The model under review builds one solid part; all positions refer to its coordinate system, in mm. Give positions to 0.01 mm unless a question says otherwise; leave off trailing zeros. Order: outer loops, then holes, each group sorted by start corner. A loop starts at its lowest first (then second) coordinate and runs counter-clockwise, first axis right, second up. Notation, with made-up numbers: (44, -1) - (99, -1) arc R9 ccw to (99, 12) - close; hole circle Ø3 at (-37.5, -21.75). An arc over 180 degrees is marked (long way). Answer as CSV lines item,"result". Start each with the question number.
Autodesk Inventor part; units mm, degrees
ref_plane "YZ Plane" through (0, 0, 0) normal (1, 0, 0) x (0, 1, 0)
ref_plane "XZ Plane" through (0, 0, 0) normal (0, 1, 0) x (-1, 0, 0)
ref_plane "XY Plane" through (0, 0, 0) normal (0, 0, 1) x (1, 0, 0)
sketch "Sketch1" plane through (0, 0, 0) normal (0, 1, 0) x (-1, 0, 0)
  circle A0 centre (0, 0) radius 3.5 construction
  line L0 (-2.0207, -3.5) -> (-4.0415, 0)
  line L1 (-4.0415, 0) -> (-2.0207, 3.5)
  line L2 (-2.0207, 3.5) -> (2.0207, 3.5)
  line L3 (2.0207, 3.5) -> (4.0415, 0)
  line L4 (4.0415, 0) -> (2.0207, -3.5)
  line L5 (2.0207, -3.5) -> (-2.0207, -3.5)
  point P0 (0, -3.5)
  dimension "d0" = 7
extrude "Extrusion1" add sketch "Sketch1" along normal mid plane 3
sketch "Sketch2" plane through (0, 1.5, 0) normal (0, 1, 0) x (1, 0, 0)
  circle A0 centre (0, 0) radius 2
  dimension "d3" = 4
extrude "Extrusion2" cut sketch "Sketch2" against normal blind 3
fillet "Fillet1" radius 0.2 12 edges at (-3.0311, 1.5, 1.75) (0, 1.5, 3.5) (3.0311, 1.5, 1.75) (3.0311, 1.5, -1.75) (0, 1.5, -3.5) (-3.0311, 1.5, -1.75) (0, -1.5, 3.5) (-3.0311, -1.5, 1.75) (-3.0311, -1.5, -1.75) (0, -1.5, -3.5) (3.0311, -1.5, -1.75) (3.0311, -1.5, 1.75)
fillet "Fillet2" radius 0.1 2 edges at (-2, 1.5, 0) (-2, -1.5, 0)
thread "Thread1"
properties part number "M4 Nut" material "Stainless Steel"
Item 1: Take a section at A-A on x = 0. Write out the cut boundary in (y, z), and give its area (3 significant figures).
Item 2: Mouldability with a two-part tool opening along X and no side actions: class faces 1 (the face through (2.993, -1.443, -1.695)), 2 (the face through (0, 0, 2)), 3 (the face through (-2, 1.5, 2)), 4 (the face through (-2.993, -1.443, 1.695)) as released by +X, released by -X, zero draft, split by the parting line, or undercut.
Item 3: Clearance check with a flat-ended pin moving along its axis: pin 1 (1.5 mm diameter, centred on x = -1, z = 0, fed in from -Y). State where the tip first meets the part, or that it passes through.
Item 4: For line 1 along Z through (x, y) = (0, -1.2); line 2 along Z through (x, y) = (-1, 1.1); line 3 along X through (y, z) = (-1.2, 0.5), list the stretches that pass through material, from the lowest coordinate up.
Item 5: Take a section at B-B on y = 0.8. Write out the cut boundary in (x, z), and give its area (3 significant figures).
Data:
1,outline,"(-1.5, -3.3) arc R0.2 ccw to (-1.3, -3.5) - (1.3, -3.5) arc R0.2 ccw to (1.5, -3.3) - (1.5, -2.1) arc R0.1 ccw to (1.4, -2) - (-1.4, -2) arc R0.1 ccw to (-1.5, -2.1) - close; (-1.5, 2.1) arc R0.1 ccw to (-1.4, 2) - (1.4, 2) arc R0.1 ccw to (1.5, 2.1) - (1.5, 3.3) arc R0.2 ccw to (1.3, 3.5) - (-1.3, 3.5) arc R0.2 ccw to (-1.5, 3.3) - close"
1,area,"8.96 mm^2"
2,face 1,"released by +X"
2,face 2,"undercut"
2,face 3,"zero draft"
2,face 4,"released by -X"
3,pin 1,"passes through"
4,line 1,"z = -3.5 to -2, 2 to 3.5"
4,line 2,"z = -3.5 to -1.73, 1.73 to 3.5"
4,line 3,"x = -3.75 to -1.94, 1.94 to 3.75"
5,outline,"(-4.04, 0) - (-2.02, -3.5) - (2.02, -3.5) - (4.04, 0) - (2.02, 3.5) - (-2.02, 3.5) - close; hole circle Ø4 at (0, 0)"
5,area,"29.9 mm^2"
